from build123d import *

# Parameters (mm, degrees)
F1_DEPTH  = 25
F2_W      = 50
F2_H      = 50
F3_DEPTH  = 900
F4_W      = 50
F4_H      = 50
F5_DEPTH  = 900
F6_W      = 180
F6_H      = 10
F7_DEPTH  = 530
F10_DEPTH = 10
F11_SIZE  = 3


with BuildPart() as f1:
    # F0 (on Top) → F1 (new body)
    with BuildSketch(Plane.XY):
        Polygon((0, 3), (3, 0), (897, 0), (900, 3), (900, 647), (897, 650), (0, 650), align=None)
    extrude(amount=F1_DEPTH)

    # F2 (on face) → F3 (join)
    with BuildSketch(Plane.XY.offset(25)):
        with Locations((675, 412.296289)):
            Rectangle(F2_W, F2_H)
    extrude(amount=F3_DEPTH)

    # F4 (on face) → F5 (join)
    with BuildSketch(Plane.XY.offset(25)):
        with Locations((325, 412.296289)):
            Rectangle(F4_W, F4_H)
    extrude(amount=F5_DEPTH)

    # F6 (on face) → F7 (join)
    with BuildSketch(Plane.XY.offset(25)):
        with Locations((500, 432.296289)):
            Rectangle(F6_W, F6_H)
    extrude(amount=F7_DEPTH)

    # F9 (on face) → F10 (join, through all)
    with BuildSketch(Plane.XZ.offset(-427.296289)):
        Polygon((410, 555), (410, 552), (413, 555), align=None)
    extrude(amount=-F10_DEPTH)

    # F11
    f11_edges = [f1.edges().sort_by_distance(p)[0] for p in [
        (410, 432.296289, 555),
        (590, 432.296289, 555),
    ]]
    chamfer(f11_edges, length=F11_SIZE)


solid = f1.part
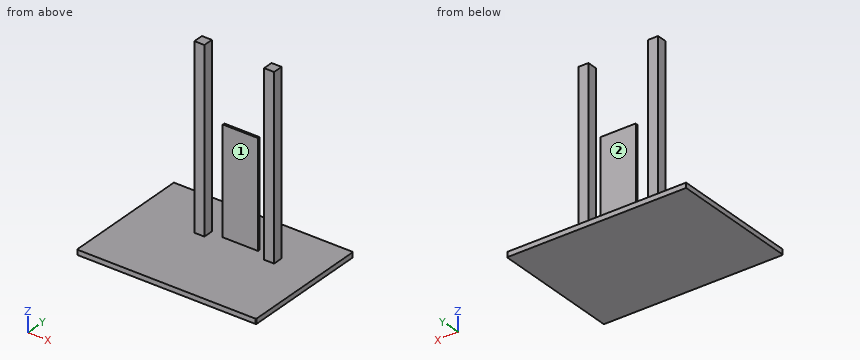
The model under review builds one solid part; all positions refer to its coordinate system, in mm. Face numbers are marked on the shaded views. Coordinates: 2 decimals unless noted, no trailing zeros. Loops run counter-clockwise (first coordinate to the right, second up) from the corner with the lowest first, then second, coordinate; pieces in that order, holes last. Notation, with made-up numbers: M 72.25,58.25 L 83.25,58.25 A30 ccw 83.25,97.25 Z; hole C 65.25,-11.75 d10. An arc over 180 degrees is marked long. Put each result on its own line as item: value. Start each with the question number.
Q1. Wall thickness on line 1 (X direction, y = 391, z = 76); line 2 (Z direction, x = 68, y = 514); line 3 (Y direction, x = 425.5, z = 554.5): over which ranges is each line inside the solid? List them lowest first.
Q2. The part is to be moulded in two halves that separate along X. For the marked faces 1 and 2, say which applies: +X half, -X half, draft (parallel to the pull), parting line (faces both ways), or undercut.
Q3. Clearance check with flat-ended pins moving along their axes: pin 1 (25 mm diameter, centred on y = 415, z = 531.5, fed in from -X); pin 2 (25 mm diameter, centred on x = 331.5, z = 314, fed in from +Y); pin 3 (4 mm diameter, centred on x = 426, z = 391, fed in from -Y); pin 4 (8 mm diameter, centred on x = 580, y = 167, fed in from -Z). State where each tip first meets the part, or that it passes through.
Q4. Add section D-D (y = 576). Write out the cut boundary in (x, z).
Q5. Add section C-C (z = 524). Write out the cut boundary in (x, y), and give its area (3 significant figures).
Q6. Add section B-B (x = 435). Write out the cut boundary in (y, z), and give its area (4 significant figures).
Q7. Add section A-A (z = 791.5). Write out the cut boundary in (x, y).
Answers:
1. line 1: x = 300 to 350, 650 to 700
1. line 2: z = 0 to 25
1. line 3: y = 427.3 to 437.3
2. face 1: undercut
2. face 2: draft
3. pin 1: stops at x = 300
3. pin 2: stops at y = 437.3
3. pin 3: stops at y = 427.3
3. pin 4: stops at z = 0
4. outline: M 0,0 L 900,0 L 900,25 L 0,25 Z
5. outline: M 300,387.3 L 350,387.3 L 350,437.3 L 300,437.3 Z; M 410,427.3 L 590,427.3 L 590,437.3 L 410,437.3 Z; M 650,387.3 L 700,387.3 L 700,437.3 L 650,437.3 Z
5. area: 6,800 mm^2
6. outline: M 0,0 L 650,0 L 650,25 L 437.3,25 L 437.3,555 L 427.3,555 L 427.3,25 L 0,25 Z
6. area: 21,550 mm^2
7. outline: M 300,387.3 L 350,387.3 L 350,437.3 L 300,437.3 Z; M 650,387.3 L 700,387.3 L 700,437.3 L 650,437.3 Z
